The listing builds one solid part. Answer for the finished solid, in the listing's coordinates (mm). Face numbers are marked on the shaded views. A direction names the side the tool comes from. Coordinates: 2 decimals unless noted, no trailing zeros. Order: outer loops, then holes, each group sorted by start corner. A loop starts at its lowest first (then second) coordinate and runs counter-clockwise, first axis right, second up.
from build123d import *

# Parameters (mm, degrees)
F0_R     = 5.08
F1_DEPTH = 50.8
F2_W     = 15.457089
F2_H     = 76.2
F3_DEPTH = 12.7
F5_D     = 6.35


with BuildPart() as f1:
    # F0 (on Front) → F1 (new body, symmetric)
    with BuildSketch(Plane.XZ):
        with BuildLine():
            ThreePointArc((8.24314, -3.175), (7.687379, -1.630541), (7.498807, 0))
            Line((7.498807, 0), (-23.457443, 0))
            Line((-23.457443, 0), (-23.457443, -3.175))
            Line((-23.457443, -3.175), (8.24314, -3.175))
        make_face()
        with BuildLine():
            ThreePointArc((8.24314, -3.175), (16.273098, -6.955178), (21.786307, 0))
            ThreePointArc((21.786307, 0), (14.642557, 7.14375), (7.498807, 0))
            ThreePointArc((7.498807, 0), (7.687379, -1.630541), (8.24314, -3.175))
        make_face()
        with Locations((14.642557, 0)):
            Circle(F0_R, mode=Mode.SUBTRACT)
    extrude(amount=F1_DEPTH, both=True)

    # F2 (on Top) → F3 (cut, symmetric)
    with BuildSketch(Plane.XY):
        with Locations((15.227614, 0)):
            Rectangle(F2_W, F2_H)
    extrude(amount=F3_DEPTH, both=True, mode=Mode.SUBTRACT)

    # F5 (through all)
    with Locations(Plane.XY):
        with Locations((-2.02593, 38.1), (-13.932443, 12.7), (-2.02593, -12.7), (-13.932443, -38.1)):
            Hole(F5_D / 2)


solid = f1.part
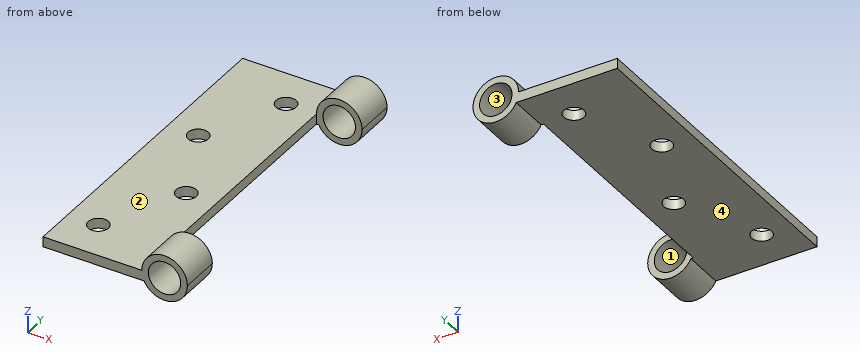
(1) Find section C-C on z = -1. Determine the outline of the cut face in (x, y) (3 decimals).
(2) Find the intervals of material crossed by probe 1 along Y at (x, z) = (14.5, -5.5); probe 2 along X at (y, z) = (-37.5, -0.25); probe 3 along Z at (x, y) = (-17, 9.5) (3 decimals), in increasing order.
(3) Given pin 1 Ø5 at (x, z) = (12.5, 4) entering from -Y; pin 2 Ø5 at (x, y) = (-17.5, -23) entering from +Z; pin 3 Ø12 at (x, y) = (-1.5, 2.5) entering from -Z (3 decimals); pin 4 Ø10 at (x, y) = (14.5, -15) entering from -Z, each flat-ended and moving along its own axis, determine where each tip first touches the part or whether it passes through.
(4) Find section D-D on x = -14. Determine the outline of the cut face in (y, z) (3 decimals).
(5) A tool of negligible diameter and unlimited length cuts with its end or side. For the marked faces 3 and 4, from which of +Z, -Z, +X, -X, +Y, -Y can it reach the whole face along a straight path? Write none if from no direction.
(6) The mould has two halves that part along X. Classify the marked faces 1 and 2: pulls with the +X half, pulls with the -X half, needs draft (parallel to the pull), parting line crosses it, or undercut.
(7) Find section B-B on x = 13.5. Determine the outline of the cut face in (y, z).
Resolved:
1. outline: (-23.457, -50.8) - (9.662, -50.8) - (9.662, -38.1) - (7.499, -38.1) - (7.499, 38.1) - (9.662, 38.1) - (9.662, 50.8) - (-23.457, 50.8) - close; (19.623, -50.8) - (21.716, -50.8) - (21.716, -38.1) - (19.623, -38.1) - close; (19.623, 38.1) - (21.716, 38.1) - (21.716, 50.8) - (19.623, 50.8) - close; hole circle Ø6.35 at (-13.932, -38.1); hole circle Ø6.35 at (-13.932, 12.7); hole circle Ø6.35 at (-2.026, -12.7); hole circle Ø6.35 at (-2.026, 38.1)
2. probe 1: y = -50.8 to -38.1, 38.1 to 50.8
2. probe 2: x = -23.46 to -17.05, -10.81 to 7.5
2. probe 3: z = -3.175 to 0
3. pin 1: stops at y = -50.8
3. pin 2: stops at z = 0
3. pin 3: stops at z = -3.175
3. pin 4: passes through
4. outline: (-50.8, -3.175) - (-41.274, -3.175) - (-41.274, 0) - (-50.8, 0) - close; (-34.926, -3.175) - (9.526, -3.175) - (9.526, 0) - (-34.926, 0) - close; (15.874, -3.175) - (50.8, -3.175) - (50.8, 0) - (15.874, 0) - close
5. face 3: +Y, -Y
5. face 4: -Z, -X, +Y, -Y
6. face 1: undercut
6. face 2: needs draft
7. outline: (-50.8, -7.05) - (-38.1, -7.05) - (-38.1, -4.95) - (-50.8, -4.95) - close; (-50.8, 4.95) - (-38.1, 4.95) - (-38.1, 7.05) - (-50.8, 7.05) - close; (38.1, -7.05) - (50.8, -7.05) - (50.8, -4.95) - (38.1, -4.95) - close; (38.1, 4.95) - (50.8, 4.95) - (50.8, 7.05) - (38.1, 7.05) - close
